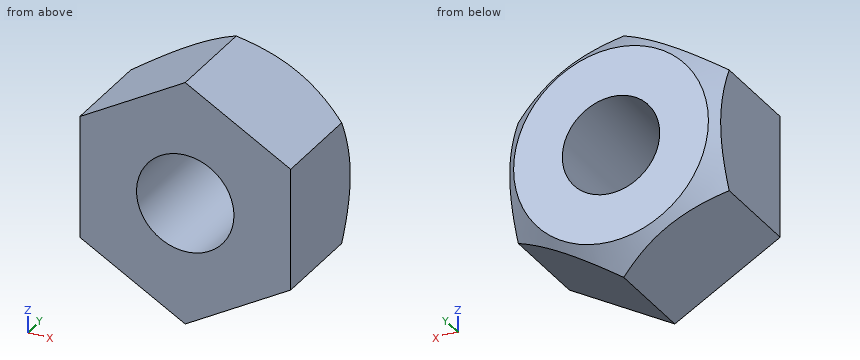
from build123d import *

# Parameters (mm, degrees)
SKETCH1_R           = 2
BOSS_EXTRUDE1_DEPTH = 5


with BuildPart() as part:
    # Sketch1 → Boss-Extrude1 (new body)
    with BuildSketch(Plane(origin=(0, 0, 0), x_dir=(1, 0, 0), z_dir=(0, 1, 0))):
        Polygon((0, 5), (-4.330127019, 2.5), (-4.330127019, -2.5), (0, -5), (4.330127019, -2.5), (4.330127019, 2.5), align=None)
        with Locations(Location((0, 0, 0), (0, 0, 270))):
            Circle(SKETCH1_R, mode=Mode.SUBTRACT)
    extrude(amount=BOSS_EXTRUDE1_DEPTH)

    # Sketch3 → Cut-Revolve1 (revolve, cut)
    with BuildSketch(Plane(origin=(0, 0, 0), x_dir=(0, 0, -1), z_dir=(1, 0, 0))):
        Polygon((4, 5), (5, 5), (5, 4), align=None)
    revolve(axis=Axis((0, 0, 0), (0, 1, 0)), mode=Mode.SUBTRACT)


solid = part.part
Verification items for the finished model (mm, model axes). Give positions to 0.01 mm unless a question says otherwise; leave off trailing zeros. Loops run counter-clockwise (first coordinate to the right, second up) from the corner with the lowest first, then second, coordinate; pieces in that order, holes last.
1. Go/stop test with flat-tipped pins: P1, Ø1, axis at x = 3, y = 4, coming from the -Z side; P2, Ø2, axis at x = -2, y = 1, coming from the +Z side; P3, Ø3.5, axis at x = 0, z = 0, coming from the -Y side. Record where each tip stops, or that it passes through.
Derived:
P1: stops at z = -3.56
P2: stops at z = 4.42
P3: passes through
2. Cross-section at A-A on z = 0. Record the cut outline in (x, y), and give its area (3 significant figures).
Derived:
outline: (-4.33, 0) - (-2, 0) - (-2, 5) - (-4, 5) - (-4.33, 4.67) - close; (2, 0) - (4.33, 0) - (4.33, 4.67) - (4, 5) - (2, 5) - close
area: 23.2 mm2
3. Material ranges on probe 1 along X at (y, z) = (3.95, 0); probe 2 along Z at (x, y) = (4.25, 4.3); probe 3 along X at (y, z) = (3.5, -0.5), recorded low to high.
Derived:
probe 1: x = -4.33 to -2, 2 to 4.33
probe 2: z = -2.01 to 2.01
probe 3: x = -4.33 to -1.94, 1.94 to 4.33
4. Cross-section at B-B on y = 2.8. Record the cut outline in (x, z), and give its area (3 significant figures).
Derived:
outline: (-4.33, -2.5) - (0, -5) - (4.33, -2.5) - (4.33, 2.5) - (0, 5) - (-4.33, 2.5) - close; hole circle Ø4 at (0, 0)
area: 52.4 mm2
